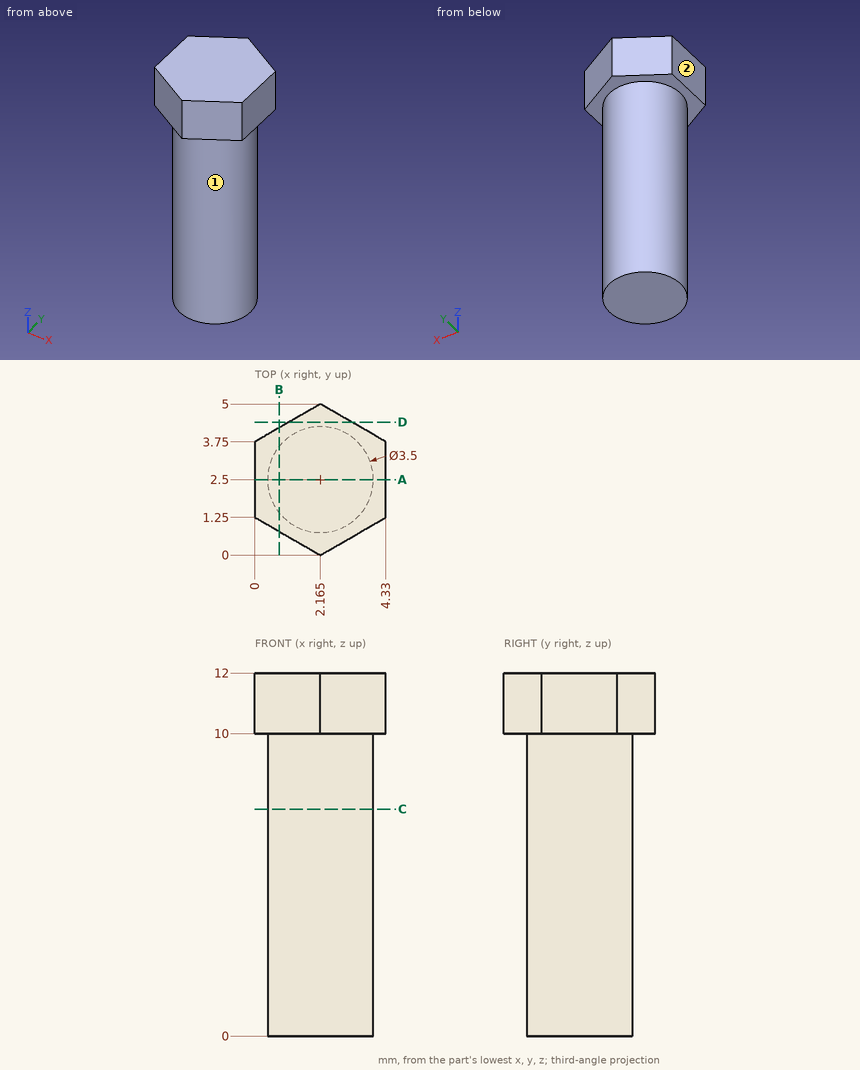
Check sheet for the drawn part. Datum: minimum x, y, z corner. Units: mm. A direction names the side the tool comes from. Coordinates: 2 decimals unless noted, no trailing zeros. Order: outer loops, then holes, each group sorted by start corner. A loop starts at its lowest first (then second) coordinate and runs counter-clockwise, first axis right, second up. Notation, with made-up numbers: (56.5, -9) - (87.5, -9) arc R25 ccw to (87.5, 7) - close; hole circle Ø7 at (4, -29). An arc over 180 degrees is marked (long way). Return JSON: item names as keys, results as strings.
(1) Access from +Z, -Z, +X, -X, +Y, -Y to the whole of each face (thin tool, end or side, straight path). Record for the marked faces 1 and 2.
Filled sheet:
{"face 1": "-Z", "face 2": "+Z, -Z, -X, +Y, -Y"}
(2) Section check A-A, the plane y = 2.5. Record the cut outline in (x, z) (3 decimals), and give its area (3 significant figures).
Filled sheet:
{"outline": "(0, 10) - (0.415, 10) - (0.415, 0) - (3.915, 0) - (3.915, 10) - (4.33, 10) - (4.33, 12) - (0, 12) - close", "area": "43.7 mm^2"}
(3) Section check B-B, the plane x = 0.8. Record the cut outline in (y, z) (3 decimals).
Filled sheet:
{"outline": "(0.788, 10) - (1.405, 10) - (1.405, 0) - (3.595, 0) - (3.595, 10) - (4.212, 10) - (4.212, 12) - (0.788, 12) - close"}
(4) Section check D-D, the plane y = 4.4. Record the cut outline in (x, z).
Filled sheet:
{"outline": "(1.13, 10) - (3.2, 10) - (3.2, 12) - (1.13, 12) - close"}
(5) Go/stop test with flat-tipped pins: pin 1 (1 mm diameter, centred on x = 3, z = 5.5, fed in from -Y); pin 2 (2 mm diameter, centred on y = 1, z = 8.5, fed in from +X). Record where each tip stops, or that it passes through.
Filled sheet:
{"pin 1": "stops at y = 0.78", "pin 2": "stops at x = 3.84"}
(6) Thickness scan on line 1 along Z through (x, y) = (3.15, 0.9); line 2 along Y through (x, z) = (3.4, 9); line 3 along X through (y, z) = (1.55, 3.5) (1 decimal). Record the ranges inside material, lowest first.
Filled sheet:
{"line 1": "z = 10 to 12", "line 2": "y = 1.26 to 3.74", "line 3": "x = 0.7 to 3.6"}
(7) Section check C-C, the plane z = 7.5. Record the cut outline in (x, y) (3 decimals).
Filled sheet:
{"outline": "circle Ø3.5 at (2.165, 2.5)"}
